Could you check a few things on this drawing? It's one solid part, dimensions in mm from its lowest x, y, z. Coordinates: 2 decimals unless noted, no trailing zeros. Order: outer loops, then holes, each group sorted by start corner. A loop starts at its lowest first (then second) coordinate and runs counter-clockwise, first axis right, second up. Notation, with made-up numbers: (4, 39) - (54, 39) arc R21 cw to (54, 48) - close; hole circle Ø1 at (43, 9). An arc over 180 degrees is marked (long way). Return JSON: item names as keys, results as strings. Group by question number.
1) If I drill on line 1 along X through (y, z) = (25.5, 0.1) (1 decimal); line 2 along Y through (x, z) = (7, 0.35); line 3 along Y through (x, z) = (42, 0.2) (1 decimal), over which ranges is the centre line in solid material (lowest first)?
2) Imagine slicing it at B-B (x = 43). Write out the boundary of the cut face in (y, z).
3) Imagine slicing it at C-C (z = 0.3). Write out the boundary of the cut face in (x, y).
4) Imagine slicing it at A-A (y = 3.9). Write out the boundary of the cut face in (x, z).
5) For pin 1 Ø4 at (x, y) = (25, 3.9) entering from +Z, with a flat end and sliding along its axis, tell me the tip position at first contact or that it passes through.
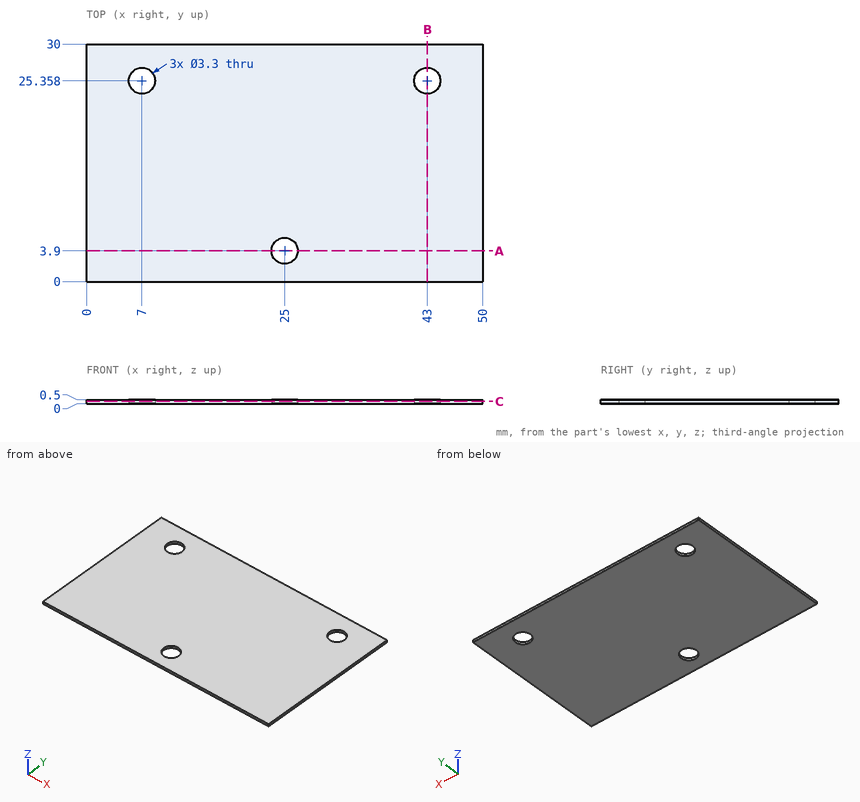
Calculated:
{
 "1": {"line 1": "0 to 5.4, 8.6 to 41.4, 44.6 to 50", "line 2": "0 to 23.71, 27.01 to 30", "line 3": "0 to 24, 26.7 to 30"},
 "2": {"outline": "(0, 0) - (23.71, 0) - (23.71, 0.5) - (0, 0.5) - close; (27.01, 0) - (30, 0) - (30, 0.5) - (27.01, 0.5) - close"},
 "3": {"outline": "(0, 0) - (50, 0) - (50, 30) - (0, 30) - close; hole circle Ø3.3 at (7, 25.36); hole circle Ø3.3 at (25, 3.9); hole circle Ø3.3 at (43, 25.36)"},
 "4": {"outline": "(0, 0) - (23.35, 0) - (23.35, 0.5) - (0, 0.5) - close; (26.65, 0) - (50, 0) - (50, 0.5) - (26.65, 0.5) - close"},
 "5": {"pin 1": "z = 0.5"}
}
